```python
from build123d import *

# Parameters (mm, degrees)
SUNGU_KIRI_R        = 1
BOSS_EXTRUDE1_DEPTH = 3
SKETCH7_R           = 7.5
CUT_EXTRUDE2_DEPTH  = 0.5
SCALE1_SCALE        = 1.75


with BuildPart() as part:
    # sungu kiri → Boss-Extrude1 (new body)
    with BuildSketch(Plane(origin=(0, 0, 0), x_dir=(1, 0, 0), z_dir=(0, 1, 0))):
        with BuildLine():
            Line((-20.214241335, 18.58200887), (-17.903708636, 25.676772527))
            Line((-17.903708636, 25.676772527), (-20.879327355, 22.419581076))
            Line((-20.879327355, 22.419581076), (-23.726014444, 13.678492013))
            ThreePointArc((-23.726014444, 13.678492013), (-25.061399851, 10.98195956), (-26.444409257, 8.309539974))
            ThreePointArc((-26.444409257, 8.309539974), (-27.383764934, 5.63006722), (-27.936945566, 2.845115782))
            ThreePointArc((-27.936945566, 2.845115782), (-28.068014235, 0.18049064), (-27.936945566, -2.484134502))
            ThreePointArc((-27.936945566, -2.484134502), (-27.425713247, -6.715299694), (-26.444409257, -10.862727794))
            ThreePointArc((-26.444409257, -10.862727794), (-25.296755437, -14.61403578), (-23.488374839, -18.095297119))
            ThreePointArc((-23.488374839, -18.095297119), (-22.238356067, -20.131176806), (-20.758136978, -22.006357992))
            ThreePointArc((-20.758136978, -22.006357992), (-13.175246696, -36.755405871), (-4.582277955, -22.571064976))
            ThreePointArc((-4.582277955, -22.571064976), (-4.460378612, -22.299351604), (-4.344569641, -22.024987085))
            ThreePointArc((-4.344569641, -22.024987085), (-4.340995805, -22.01171692), (-4.3373846, -21.998456875))
            ThreePointArc((-4.3373846, -21.998456875), (-4.667057778, -21.129677391), (-5.155481579, -20.33916845))
            ThreePointArc((-5.155481579, -20.33916845), (-7.110923153, -19.117606911), (-9.361873626, -18.618421268))
            ThreePointArc((-9.361873626, -18.618421268), (-11.285784226, -18.376920372), (-13.150188878, -17.844238508))
            ThreePointArc((-13.150188878, -17.844238508), (-15.818147575, -16.60648921), (-18.010368345, -14.645827324))
            ThreePointArc((-18.010368345, -14.645827324), (-20.650416196, -11.005311906), (-22.72256926, -7.01414831))
            ThreePointArc((-22.72256926, -7.01414831), (-21.584958488, 10.98418111), (-6.423603233, 20.74980075))
            Line((-6.423603233, 20.74980075), (-7.667855794, 21.470443038))
            Line((-7.667855794, 21.470443038), (-16.17291449, 19.521519125))
            Line((-16.17291449, 19.521519125), (-20.214241335, 16.223172594))
            Line((-20.214241335, 16.223172594), (-20.214241335, 18.58200887))
        make_face()
        with Locations(Location((-12.843799059, -27.261189607, 0), (0, 0, 270))):
            Circle(SUNGU_KIRI_R, mode=Mode.SUBTRACT)
    extrude(amount=BOSS_EXTRUDE1_DEPTH)

    # Sketch7 → Cut-Extrude2 (cut)
    with BuildSketch(Plane(origin=(0, 0, 0), x_dir=(1, 0, 0), z_dir=(0, 1, 0))):
        with Locations(Location((-12.843799059, -27.261189607, 0), (0, 0, 270))):
            Circle(SKETCH7_R)
    extrude(amount=CUT_EXTRUDE2_DEPTH, mode=Mode.SUBTRACT)


with BuildPart() as part_1:
    # Scale1: scaled about (-17.083309672, 1.577817205, 15.178250086)
    add(part.part.scale(SCALE1_SCALE).moved(Location((12.812482254, -1.183362904, -11.383687565))))


solid = part_1.part
```
Verification items for the finished model (mm, model axes). A direction names the side the tool comes from. Give positions to 0.01 mm unless a question says otherwise; leave off trailing zeros. Order: outer loops, then holes, each group sorted by start corner. A loop starts at its lowest first (then second) coordinate and runs counter-clockwise, first axis right, second up. Notation, with made-up numbers: M 78,-27.75 L 128,-27.75 A19 cw 128,-15.75 Z; hole C 76,83.25 d4. An arc over 180 degrees is marked long. Return JSON: item names as keys, results as strings. Group by question number.
1) Go/stop test with flat-tipped pins: pin 1 Ø16 at (x, z) = (-9.66, 36.32) entering from +Y; pin 2 Ø2 at (y, z) = (2.5, 23.5) entering from -X; pin 3 Ø3 at (x, z) = (-9.66, 36.32) entering from +Y (3 decimals); pin 4 Ø3 at (x, y) = (-11.5, 2.5) entering from -Z. Record where each tip stops, or that it passes through.
2) Scan lines: line 1 (Z direction, x = -2, y = 2.35); line 2 (Y direction, x = -13.5, z = 33.5); line 3 (X direction, y = -0.3, z = -43). Record each from-to range of solid material in increasing order.
3) Mould release check, pull along Z, two halves, no side actions. Record for faces 1 (the face through (-18, 4.067, 18)), 2 (the face through (-14.809, 1.405, 17.717)), 3 (the face through (-35.2, 1.4, 0.27)): pulls with the +Z half, pulls with the -Z half, needs draft (parallel to the pull), parting line crosses it, or undercut.
4) Section check C-C on z = 26. Record the cut outline in (x, y).
5) Access from +Z, -Z, +X, -X, +Y, -Y to the whole of each face (thin tool, end or side, straight path). Record for faces 4 (the face through (-6.891, 1.405, 20.785)), 5 (the face through (-26.138, 1.405, 23.798)), 6 (the face through (-35.09, 1.4, -21.3)), 7 (the face through (-9, -0.308, 39)), 8 (the face through (-18.98, 1.4, -42.7)).
6) Section check A-A on x = -6. Record the cut outline in (y, z), and give its area (3 significant figures).
7) Section check D-D on x = -16.5. Record the cut outline in (y, z), and give its area (3 significant figures).
Answer block:
{
 "1": {"pin 1": "stops at y = 4.07", "pin 2": "stops at x = -27", "pin 3": "passes through", "pin 4": "stops at z = -46.8"},
 "2": {"line 1": "z = -48.64 to -47.13, 21.38 to 51.08", "line 2": "y = -0.31 to 4.07", "line 3": "x = -26.21 to -22.56, -18.61 to -12.62"},
 "3": {"face 1": "needs draft", "face 2": "undercut", "face 3": "pulls with the +Z half"},
 "4": {"outline": "M -24.48,-1.18 L -17.77,-1.18 L -17.77,-0.31 L -1.56,-0.31 L -1.56,-1.18 L 4.83,-1.18 L 4.83,4.07 L -24.48,4.07 Z"},
 "5": {"face 4": "+X, +Y, -Y", "face 5": "-X, +Y, -Y", "face 6": "-Z, -X, +Y, -Y", "face 7": "-Y", "face 8": "+Y, -Y"},
 "6": {"outline": "M -1.18,-47.72 L 4.07,-47.72 L 4.07,-46.04 L -1.18,-46.04 Z; M -1.18,20.95 L 4.07,20.95 L 4.07,52.54 L -1.18,52.54 L -1.18,48.93 L -0.31,48.93 L -0.31,23.72 L -1.18,23.72 Z", "area": "153 mm^2"},
 "7": {"outline": "M -1.18,-44.72 L 4.07,-44.72 L 4.07,-40.33 L -1.18,-40.33 Z; M -1.18,16.46 L 4.07,16.46 L 4.07,51.48 L -1.18,51.48 L -1.18,47.53 L -0.31,47.53 L -0.31,25.12 L -1.18,25.12 Z", "area": "187 mm^2"}
}
